Geometry check sheet. Reference: the model listing, model coordinates, mm. A direction names the side the tool comes from. Give positions to 0.01 mm unless a question says otherwise; leave off trailing zeros. Loops run counter-clockwise (first coordinate to the right, second up) from the corner with the lowest first, then second, coordinate; pieces in that order, holes last. Notation, with made-up numbers: (-33.75, -19) -> (-18.75, -19) arc R12 cw to (-18.75, -14) -> close; hole circle Ø7 at (66, 64). An arc over 180 degrees is marked (long way). One line per item, written item: value. Start each with the question number.
(1) Draft check along X on faces 3 (the face through (116.975, 1426.494, -190.477)), 4 (the face through (-155.575, 1433, -190)), 5 (the face through (222.25, 1433, -190)), 6 (the face through (219.119, 1413.806, -191.035)). Enter one of: pulls with the +X half, pulls with the -X half, needs draft (parallel to the pull), parting line crosses it, or undercut.
(2) Sectioned sample at A-A, the plane x = -95. Record the cut outline in (y, z).
(3) Scan lines: line 1 along X through (y, z) = (1434.5, -199.5) (3 decimals); line 2 along X through (y, z) = (1434, -178) (3 decimals); line 3 along X through (y, z) = (1423, -181.5) (3 decimals). Record each from-to range of solid material in increasing order. Write a range as from..to.
(4) Gauge pin test, flat ends, axial feed: pin 1 Ø6 at (x, y) = (-25.5, 1441) entering from +Z; pin 2 Ø1 at (x, z) = (176.5, -196.5) entering from -Y; pin 3 Ø1 at (x, y) = (145, 1438) entering from -Z. Record the tip position at first contact, or that the pin passes through.
(5) Tool access check on faces 1 (the face through (-152.713, 1413.806, -191.035)), 2 (the face through (15.24, 1427, -193.2)). Record the directions out of +Z, -Z, +X, -X, +Y, -Y that give a thin tool (end or side, any length) a straight path to the whole face; none if there is none.
from build123d import *

# Parameters (mm, degrees)
SKETCH3_R = 0.635


with BuildPart() as part:
    # Sketch2 → Revolve1 (revolve)
    with BuildSketch(Plane(origin=(25.4, 0, -190.199803954), x_dir=(1, 0, 0), z_dir=(0, 0, 1))):
        with BuildLine():
            Line((-10.16, 1439.086510137), (114.3, 1439.086510137))
            Line((114.3, 1439.086510137), (190.5, 1439.086510137))
            Line((190.5, 1439.086510137), (190.5, 1451.786510137))
            Line((190.5, 1451.786510137), (196.85, 1451.786510137))
            Line((196.85, 1451.786510137), (196.85, 1432.787310137))
            Line((196.85, 1432.787310137), (-180.975, 1432.787310137))
            Line((-180.975, 1432.787310137), (-180.975, 1449.246510137))
            ThreePointArc((-180.975, 1449.246510137), (-180.231051224, 1451.042561361), (-178.435, 1451.786510137))
            Line((-178.435, 1451.786510137), (-177.8, 1451.786510137))
            Line((-177.8, 1451.786510137), (-177.8, 1439.086510137))
            Line((-177.8, 1439.086510137), (-101.6, 1439.086510137))
            Line((-101.6, 1439.086510137), (-91.44, 1439.086510137))
            Line((-91.44, 1439.086510137), (-22.86, 1439.086510137))
            Line((-22.86, 1439.086510137), (-22.86, 1445.334910137))
            Line((-22.86, 1445.334910137), (-10.16, 1445.334910137))
            Line((-10.16, 1445.334910137), (-10.16, 1439.086510137))
        make_face()
    revolve(axis=Axis((25.4, 1432.787310137, -190.199803954), (-1, 0, 0)))

    # Sketch3 → Cut-Revolve1 (revolve, cut)
    with BuildSketch(Plane(origin=(25.4, 0, -190.199803954), x_dir=(1, 0, 0), z_dir=(0, 0, 1))):
        with Locations((-16.51, 1445.334910137)):
            Circle(SKETCH3_R)
    revolve(axis=Axis((2.54, 1432.787310137, -190.199803954), (1, 0, 0)), mode=Mode.SUBTRACT)


solid = part.part
Calculated:
1. face 3: undercut
1. face 4: pulls with the -X half
1. face 5: pulls with the +X half
1. face 6: needs draft
2. outline: circle Ø12.6 at (1432.79, -190.2)
3. line 1: x = -155.575..-152.4, 2.54..15.24, 215.9..222.25
3. line 2: x = -155.575..-152.4, 2.54..8.324, 9.456..15.24, 215.9..222.25
3. line 3: x = -155.575..-152.4, 215.9..222.25
4. pin 1: stops at z = -186.66
4. pin 2: stops at y = 1430.33
4. pin 3: stops at z = -194.38
5. face 1: +X, -X
5. face 2: none
